Check sheet for the modelled part. Datum: model origin and axes. Units: mm. Face numbers are marked on the shaded views. A direction names the side the tool comes from. Round coordinates to 2 decimals unless told otherwise and drop trailing zeros. Order: outer loops, then holes, each group sorted by start corner. A loop starts at its lowest first (then second) coordinate and runs counter-clockwise, first axis right, second up.
(1) Thickness scan on probe 1 along Z at (x, y) = (41, -42) (3 decimals); probe 2 along X at (y, z) = (12.5, 4.5) (3 decimals); probe 3 along Z at (x, y) = (94, 16). Record the ranges inside material, lowest first.
(2) Tool access check on the marked faces 1, 2, 3, 4 and 5. Record the directions out of +Z, -Z, +X, -X, +Y, -Y that give a thin tool (end or side, any length) a straight path to the whole face; none if there is none.
(3) Depth check by flat-ended pin: pin 1 (2 mm diameter, centred on x = 34.5, z = 26, fed in from +Y); pin 2 (12 mm diameter, centred on x = 10, z = 51, fed in from -Y); pin 3 (5 mm diameter, centred on y = -15, z = 19, fed in from -X). Enter the tip coordinate at first touch or a pass-through.
(4) Sectioned sample at B-B, the plane x = 61.5. Enter the section's corners in (y, z).
(5) Sectioned sample at A-A, the plane y = 11.5. Enter the section's corners in (x, z) (3 decimals).
(6) Sectioned sample at C-C, the plane y = -47. Enter the section's corners in (x, z) (3 decimals), and give its area (3 significant figures).
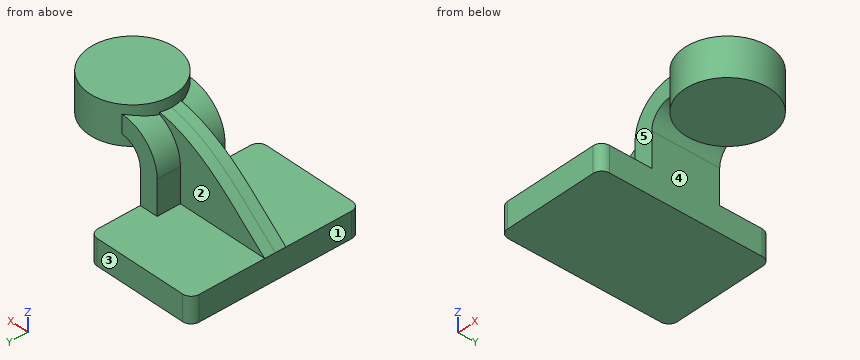
```python
from build123d import *

# Parameters (mm, degrees)
F1_DEPTH = 63.5
F2_DEPTH = 7.9375
F3_DEPTH = 25.4
F4_R     = 6.35


# Not quite as in the source:
# - ends of sketch curves that miss each other by under 0.0002 mm in the source are joined


with BuildPart() as f1:
    # F0 (on Front) → F1 (new body, symmetric)
    with BuildSketch(Plane.XZ):
        Polygon((-41.275, 9.525), (-41.275, -9.525), (41.275, -9.525), (41.275, 9.525), (27.5589991361, 9.525), align=None)
    extrude(amount=F1_DEPTH, both=True)

    # F0 (on Front) → F2 (join, symmetric)
    with BuildSketch(Plane.XZ):
        with BuildLine():
            add(Edge.make_bspline(
                [(-41.275, 9.525), (-12.8610799571, 32.6827113613), (12.6950968294, 62.5117734864), (54.8244975817, 64.1265564996)],
                knots=[0, 0, 0, 0, 110.5540678871, 110.5540678871, 110.5540678871, 110.5540678871], degree=3))
            Line((-41.275, 9.525), (27.5589991361, 9.525))
            Line((27.5589991361, 9.525), (27.5589991361, 35.2199450135))
            ThreePointArc((27.5589991361, 35.2199450135), (35.450810299, 55.0882589398), (54.8244975817, 64.1265564996))
        make_face()
    extrude(amount=F2_DEPTH, both=True)

    # F0 (on Front) → F3 (join, symmetric)
    with BuildSketch(Plane.XZ):
        with BuildLine():
            Line((27.5589991361, 9.525), (41.275, 9.525))
            Line((41.275, 9.525), (41.275, 35.2199450135))
            ThreePointArc((41.275, 35.2199450135), (45.7386926547, 45.9962523588), (56.515, 50.4599450135))
            Line((56.515, 50.4599450135), (56.515, 64.1759467518))
            add(Edge.make_bspline(
                [(54.8244975817, 64.1265564996), (55.3850490812, 64.1480419473), (55.9485346305, 64.1645324648), (56.515, 64.1759467518)],
                knots=[110.5540678871, 110.5540678871, 110.5540678871, 110.5540678871, 112.0250417777, 112.0250417777, 112.0250417777, 112.0250417777], degree=3))
            ThreePointArc((54.8244975817, 64.1265564996), (35.450810299, 55.0882589398), (27.5589991361, 35.2199450135))
            Line((27.5589991361, 35.2199450135), (27.5589991361, 9.525))
        make_face()
    extrude(amount=F3_DEPTH, both=True)

    # F4
    f4_edges = [f1.edges().sort_by_distance(p)[0] for p in [
        (-41.275, -63.5, 0),
        (41.275, -63.5, 0),
        (41.275, 63.5, 0),
        (-41.275, 63.5, 0),
    ]]
    fillet(f4_edges, radius=F4_R)

    # F0 (on Front) → F5 (revolve)
    with BuildSketch(Plane.XZ):
        Polygon((75.4097700119, 70.9069057465), (75.4097700119, 64.1759485006), (75.4097700119, 50.4599450135), (75.4097700119, 42.3319057465), (107.315, 42.3319057465), (107.315, 70.9069057465), align=None)
    revolve(axis=Axis((75.4097700119, 0, 56.6194057465), (0, 0, 1)))


solid = f1.part
```
Derived:
1. probe 1: z = -9.525 to 9.525
1. probe 2: x = -41.275 to 41.275
1. probe 3: z = 42.33 to 70.91
2. face 1: +Z, -Z, -X, +Y, -Y
2. face 2: +Z, -X, +Y
2. face 3: +Z, -Z, +X, -X, +Y
2. face 4: -Z, +X, +Y, -Y
2. face 5: +Z, -X, -Y
3. pin 1: stops at y = 25.4
3. pin 2: stops at y = -7.94
3. pin 3: stops at x = 27.56
4. outline: (-28.71, 42.33) - (28.71, 42.33) - (28.71, 70.91) - (-28.71, 70.91) - close
5. outline: (-41.275, -9.525) - (41.275, -9.525) - (41.275, 35.22) arc R15.24 cw to (45.649, 45.906) - (45.649, 42.332) - (105.17, 42.332) - (105.17, 70.907) - (45.649, 70.907) - (45.649, 62.06) arc R28.956 ccw to (27.559, 35.22) - (27.559, 9.525) - (-41.275, 9.525) - close
6. outline: (-41.275, -9.525) - (41.275, -9.525) - (41.275, 9.525) - (-41.275, 9.525) - close
6. area: 1,570 mm2
